```python
from build123d import *

# Parameters (mm, degrees)
F0_W     = 76.2
F0_H     = 76.2
F1_DEPTH = 76.2
F2_W     = 25.4
F2_H     = 25.4
F3_DEPTH = 12.7
F5_D     = 25.4
F6_R     = 12.7
F7_DEPTH = 12.7
F8_SIZE  = 5.08
F9_SIZE  = 5.08
F10_SIZE = 5.08
F11_SIZE = 5.08
F12_SIZE = 5.08
F13_SIZE = 5.08
F14_SIZE = 5.08
F15_SIZE = 5.08
F16_SIZE = 5.08
F17_SIZE = 5.08


# Not quite as in the source:
# - the program builds the solid bodies; features that only make, move or delete a surface that nothing else refers to are left out


with BuildPart() as f1:
    # F0 (on Front) → F1 (new body)
    with BuildSketch(Plane.XZ):
        with Locations((-38.1, 38.1)):
            Rectangle(F0_W, F0_H)
    extrude(amount=F1_DEPTH)

    # F2 (on face) → F3 (join)
    with BuildSketch(Plane.XZ.offset(76.2)):
        with Locations((-38.1, 38.1)):
            Rectangle(F2_W, F2_H)
    extrude(amount=F3_DEPTH)

    # F5 (through all)
    with Locations(Plane.XY.offset(76.2)):
        with Locations((-38.1, -38.1)):
            Hole(F5_D / 2)

    # F6 (on face) → F7 (join)
    with BuildSketch(Plane.YZ):
        with Locations((-38.1, 38.1)):
            Circle(F6_R)
    extrude(amount=F7_DEPTH)

    # F8
    f8_edges = [f1.edges().sort_by_distance(p)[0] for p in [
        (-38.1, -76.2, 76.2),
        (0, -38.1, 76.2),
    ]]
    chamfer(f8_edges, length=F8_SIZE)

    # F9
    f9_edges = [f1.edges().sort_by_distance(p)[0] for p in [
        (-40.64, 0, 76.2),
    ]]
    chamfer(f9_edges, length=F9_SIZE)

    # F10
    f10_edges = [f1.edges().sort_by_distance(p)[0] for p in [
        (-76.2, -38.1, 76.2),
    ]]
    chamfer(f10_edges, length=F10_SIZE)

    # F11
    f11_edges = [f1.edges().sort_by_distance(p)[0] for p in [
        (0, -76.2, 35.56),
        (-76.2, -76.2, 35.56),
    ]]
    chamfer(f11_edges, length=F11_SIZE)

    # F12
    f12_edges = [f1.edges().sort_by_distance(p)[0] for p in [
        (-38.1, -76.2, 0),
    ]]
    chamfer(f12_edges, length=F12_SIZE)

    # F13
    f13_edges = [f1.edges().sort_by_distance(p)[0] for p in [
        (0, -35.56, 0),
    ]]
    chamfer(f13_edges, length=F13_SIZE)

    # F14
    f14_edges = [f1.edges().sort_by_distance(p)[0] for p in [
        (0, 0, 38.1),
    ]]
    chamfer(f14_edges, length=F14_SIZE)

    # F15
    f15_edges = [f1.edges().sort_by_distance(p)[0] for p in [
        (-76.2, 0, 35.56),
    ]]
    chamfer(f15_edges, length=F15_SIZE)

    # F16
    f16_edges = [f1.edges().sort_by_distance(p)[0] for p in [
        (-76.2, -38.1, 0),
    ]]
    chamfer(f16_edges, length=F16_SIZE)

    # F17
    f17_edges = [f1.edges().sort_by_distance(p)[0] for p in [
        (-38.1, 0, 0),
    ]]
    chamfer(f17_edges, length=F17_SIZE)


solid = f1.part
```
Here's how the part is built. I have some questions about the finished solid (model axes, mm). A direction names the side the tool comes from. Give positions to 0.01 mm unless a question says otherwise; leave off trailing zeros. Order: outer loops, then holes, each group sorted by start corner. A loop starts at its lowest first (then second) coordinate and runs counter-clockwise, first axis right, second up. Notation, with made-up numbers: (19, 86) -> (43, 86) arc R33 ccw to (43, 119) -> close; hole circle Ø4 at (65, 42.25). An arc over 180 degrees is marked (long way). Use CSV: the item, a comma, the result in double quotes. Start each with the question number.
Item 1: Suppose I cut it at D-D (y = -67). List the corners of the cut face in (x, z) for me.
Item 2: I'm going to push flat-ended pins straight in: P1, Ø5, axis at y = -65.5, z = 55, coming from the +X side; P2, Ø14, axis at x = -36.5, y = -85, coming from the +Z side; P3, Ø6.5, axis at y = -84, z = 40.5, coming from the +X side. Where does each tip first touch, or does it pass through?
Item 3: Suppose I cut it at B-B (z = 64). List the corners of the cut face in (x, y) for me.
Item 4: Thinking about a two-plate mould opening in Z: for faces 5 (the flat face through (-2.5, -37.6, 2.58)), 6 (the flat face through (12.7, -38, 38)), 7 (the flat face through (-2.5, -37.6, 73.62)), which applies, pulls with the +Z half, pulls with the -Z half, needs draft (parallel to the pull), parting line crosses it, or undercut?
Item 5: If I drill on probe 1 along Y at (x, z) = (-38, 21); probe 2 along Y at (x, z) = (-38, 35); probe 3 along X at (y, z) = (-59, 28.5), over which ranges is the centre line in solid material (lowest first)? Write a range as [from, to].
Item 6: Suppose I cut it at C-C (y = -38.1). List the corners of the cut face in (x, z) for me.
Item 7: Suppose I cut it at A-A (x = -38.1). List the corners of the cut face in (y, z) for me, and give its area (3 significant figures).
Item 8: On a 3-axis mill with a long thin cutter (end or side, diameter ignored), from which of +Z, -Z, +X, -X, +Y, -Y can I reach the whole of each face in a straight line? I mean faces 1 (the flat face through (0, -52, 38)), 2 (the flat face through (-25.4, -82, 38)), 3 (the flat face through (-50.8, -82, 38)), 4 (the flat face through (-38.6, -73.7, 2.58)). Say none if no direction works.
Answer block:
1,outline,"(-76.2, 5.08) -> (-71.12, 0) -> (-5.08, 0) -> (0, 5.08) -> (0, 71.12) -> (-5.08, 76.2) -> (-71.12, 76.2) -> (-76.2, 71.12) -> close"
2,P1,"stops at x = 0"
2,P2,"stops at z = 50.8"
2,P3,"stops at x = -25.4"
3,outline,"(-76.2, -71.12) -> (-71.12, -76.2) -> (-5.08, -76.2) -> (0, -71.12) -> (0, -5.08) -> (-5.08, 0) -> (-71.12, 0) -> (-76.2, -5.08) -> close; hole circle Ø25.4 at (-38.1, -38.1)"
4,face 5,"pulls with the -Z half"
4,face 6,"needs draft"
4,face 7,"pulls with the +Z half"
5,probe 1,"y = [-76.2, -50.8], [-25.4, 0]"
5,probe 2,"y = [-88.9, -50.8], [-25.4, 0]"
5,probe 3,"x = [-76.2, 0]"
6,outline,"(-76.2, 5.08) -> (-71.12, 0) -> (-50.8, 0) -> (-50.8, 76.2) -> (-71.12, 76.2) -> (-76.2, 71.12) -> close; (-25.4, 0) -> (-5.08, 0) -> (0, 5.08) -> (0, 25.4) -> (12.7, 25.4) -> (12.7, 50.8) -> (0, 50.8) -> (0, 71.12) -> (-5.08, 76.2) -> (-25.4, 76.2) -> close"
7,outline,"(-88.9, 25.4) -> (-76.2, 25.4) -> (-76.2, 5.08) -> (-71.12, 0) -> (-50.8, 0) -> (-50.8, 76.2) -> (-71.12, 76.2) -> (-76.2, 71.12) -> (-76.2, 50.8) -> (-88.9, 50.8) -> close; (-25.4, 0) -> (-5.08, 0) -> (0, 5.08) -> (0, 71.12) -> (-5.08, 76.2) -> (-25.4, 76.2) -> close"
7,area,"4,140 mm^2"
8,face 1,"+X"
8,face 2,"+Z, -Z, +X, -Y"
8,face 3,"+Z, -Z, -X, -Y"
8,face 4,"-Z, +X, -X, -Y"
